The listing builds one solid part. Answer for the finished solid, in the listing's coordinates (mm). Face numbers are marked on the shaded views. Give positions to 0.01 mm unless a question says otherwise; leave off trailing zeros. Write each loop counter-clockwise with the first axis right and the second up, starting at its lowest first coordinate (ties: lowest second). Pieces come first, ordered by that corner, then holes. Notation, with made-up numbers: (23.5, 76) - (54.5, 76) arc R37 cw to (54.5, 114) - close; hole circle Ø7 at (41.5, 67.25). An arc over 180 degrees is marked (long way). One line per question, with ' | ' between items. Start each with the question number.
1. The mould has two halves that part along Z. Classify the marked faces 1, 2 and 3: +Z half, -Z half, draft (parallel to the pull), parting line (faces both ways), or undercut.
2. Find the intervals of material crossed by L1, parallel to Y at x = 25.5, z = 3.5; L2, parallel to Y at x = 82.5, z = 6.25; L3, parallel to X at y = -30, z = 1.5, in increasing order. Write a range as from..to.
3. Given P1, Ø1.5, axis at x = -80, y = 7.5, coming from the -Z side; P2, Ø0.9, axis at y = 0, z = 7.5, coming from the -X side; P3, Ø1.5, axis at y = -20.5, z = 8, coming from the +X side; P4, Ø1.5, axis at y = -3, z = 2, coming from the +X side, each flat-ended and moving along its own axis, determine where each tip first touches the part or whether it passes through.
4. A cutting plane is placed at B-B (y = -27.5). Determine the outline of the cut face in (x, z).
5. A cutting plane is placed at A-A (x = -20.5). Determine the outline of the cut face in (y, z).
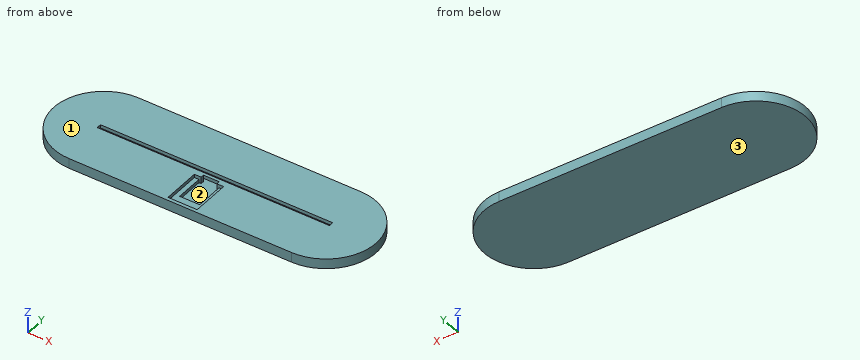
```python
from build123d import *

# Parameters (mm, degrees)
PAD_DEPTH       = 3
PAD001_DEPTH    = 3
SKETCH002_W     = 209.08447
SKETCH002_H     = 4.18
PAD002_DEPTH    = 3
SKETCH003_W     = 26.3
SKETCH003_H     = 34.2
POCKET_DEPTH    = 3
SKETCH004_W     = 18
SKETCH004_H     = 25
POCKET001_DEPTH = 3
SKETCH005_W     = 14
SKETCH005_H     = 3
POCKET002_DEPTH = 6


with BuildPart() as part:
    # Sketch → Pad (new body)
    with BuildSketch(Plane.XY):
        with BuildLine():
            ThreePointArc((-100, 45), (-145, 0), (-100, -45))
            Line((-100, -45), (100, -45))
            ThreePointArc((100, -45), (145, 0), (100, 45))
            Line((-100, 45), (100, 45))
        make_face()
    extrude(amount=PAD_DEPTH)

    # Sketch001 (on Face6 of Pad) → Pad001 (join)
    with BuildSketch(Plane.XY.offset(3)):
        with BuildLine():
            ThreePointArc((-100, 45), (-145, 0), (-100, -45))
            Line((-100, -45), (100, -45))
            ThreePointArc((100, -45), (145, 0), (100, 45))
            Line((-100, 45), (100, 45))
        make_face()
        with BuildLine():
            ThreePointArc((-100, 5), (-105, 0), (-100, -5))
            Line((-100, -5), (100, -5))
            ThreePointArc((100, -5), (105, 0), (100, 5))
            Line((-100, 5), (100, 5))
        make_face(mode=Mode.SUBTRACT)
    extrude(amount=PAD001_DEPTH)

    # Sketch002 (on Face9 of Pad001) → Pad002 (join)
    with BuildSketch(Plane.XY.offset(6)):
        with BuildLine():
            ThreePointArc((-100, 45), (-145, 0), (-100, -45))
            Line((-100, -45), (100, -45))
            ThreePointArc((100, -45), (145, 0), (100, 45))
            Line((-100, 45), (100, 45))
        make_face()
        Rectangle(SKETCH002_W, SKETCH002_H, mode=Mode.SUBTRACT)
    extrude(amount=PAD002_DEPTH)

    # Sketch003 (on Face13 of Pad002) → Pocket (cut)
    with BuildSketch(Plane.XY.offset(9)):
        with Locations((0, -24.9)):
            Rectangle(SKETCH003_W, SKETCH003_H)
    extrude(amount=-POCKET_DEPTH, mode=Mode.SUBTRACT)

    # Sketch004 (on Face27 of Pocket) → Pocket001 (cut)
    with BuildSketch(Plane.XY.offset(6)):
        with Locations((0, -20.3)):
            Rectangle(SKETCH004_W, SKETCH004_H)
    extrude(amount=-POCKET001_DEPTH, mode=Mode.SUBTRACT)

    # Sketch005 (on Face13 of Pocket001) → Pocket002 (cut)
    with BuildSketch(Plane.XY.offset(9)):
        with Locations((0, -6.3)):
            Rectangle(SKETCH005_W, SKETCH005_H)
    extrude(amount=-POCKET002_DEPTH, mode=Mode.SUBTRACT)


solid = part.part
```
Determined:
1) face 1: +Z half | face 2: undercut | face 3: -Z half
2) L1: -45..-5, 5..45 | L2: -45..-2.09, 2.09..45 | L3: -133.54..133.54
3) P1: z = 0 | P2: x = -145 | P3: x = 140.43 | P4: x = 144.94
4) outline: (-135.62, 0) - (135.62, 0) - (135.62, 9) - (13.15, 9) - (13.15, 6) - (9, 6) - (9, 3) - (-9, 3) - (-9, 6) - (-13.15, 6) - (-13.15, 9) - (-135.62, 9) - close
5) outline: (-45, 0) - (45, 0) - (45, 9) - (2.09, 9) - (2.09, 6) - (5, 6) - (5, 3) - (-5, 3) - (-5, 6) - (-2.09, 6) - (-2.09, 9) - (-45, 9) - close
